Autodesk Inventor part; units mm, degrees
ref_plane "Start Plane" through (0, 0, 0) normal (1, 0, 0) x (0, 1, 0)
ref_plane "XZ Plane" through (0, 0, 0) normal (0, 1, 0) x (-1, 0, 0)
ref_plane "XY Plane" through (0, 0, 0) normal (0, 0, 1) x (1, 0, 0)
sketch "Main Sketch" plane through (0, 0, 0) normal (0, 0, 1) x (1, 0, 0)
  line L0 (0, 0) -> (40, 0)
  line L1 (0, 3) -> (0, 10)
  line L2 (40, 10) -> (40, 3)
  line L3 (0, 10) -> (40, 10)
  line L4 (12, 3) -> (12, 0)
  line L5 (0, 3) -> (12, 3)
  line L6 (28, 3) -> (28, 0)
  line L7 (40, 3) -> (28, 3)
  line L8 (12, 0) -> (28, 0)
  dimension "d3" = 20
  dimension "d4" = 6
  dimension "d5" = 6
revolve "Revolution1" add sketch "Main Sketch" angle 360 about axis through (0, 0, 0) along (1, 0, 0)
equation "\"Length\" = 40"
properties part number "Shaft" material "Aluminum 6061"
Check sheet for the modelled part. Datum: model origin and axes. Units: mm. A direction names the side the tool comes from. Coordinates: 2 decimals unless noted, no trailing zeros. Write each loop counter-clockwise with the first axis right and the second up, starting at its lowest first coordinate (ties: lowest second). Pieces come first, ordered by that corner, then holes. Notation, with made-up numbers: M 50,59 L 69,59 A9 ccw 69,68 Z; hole C 87.25,31.5 d6. An arc over 180 degrees is marked long. Answer as CSV lines item,"result".
Q1. Set-up check for faces 5 (the face through (12, 0, 0)), 6 (the face through (0, 2.1, 2.4)), 7 (the face through (28, 0, 0)): record each of +Z, -Z, +X, -X, +Y, -Y from which the full face is reachable in a straight line by a thin tool's end or side.
Check result:
face 5,"-X"
face 6,"+Z, -Z, -X, +Y, -Y"
face 7,"+X"
Q2. Mould release check, pull along Y, two halves, no side actions. Record for faces 1 (the face through (40, 2.1, 2.4)), 2 (the face through (20.28, -2.17, -9.76)), 3 (the face through (34, -3, 0)), 4 (the face through (6, -3, 0)): released by +Y, released by -Y, zero draft, split by the parting line, or undercut.
Check result:
face 1,"zero draft"
face 2,"split by the parting line"
face 3,"undercut"
face 4,"undercut"
Q3. Cross-section at C-C (x = 27.5). Record the boundary of the cut face in (y, z).
Check result:
outline,"C 0,0 d20"
Q4. Cross-section at D-D (x = 2). Record the boundary of the cut face in (y, z), then the cut area to 3 significant figures.
Check result:
outline,"C 0,0 d20; hole C 0,0 d6"
area,"286 mm^2"
Q5. Cross-section at A-A (z = 0). Record the boundary of the cut face in (x, y), then the cut area to 3 significant figures.
Check result:
outline,"M 0,-10 L 40,-10 L 40,-3 L 28,-3 L 28,3 L 40,3 L 40,10 L 0,10 L 0,3 L 12,3 L 12,-3 L 0,-3 Z"
area,"656 mm^2"
Q6. Go/stop test with flat-tipped pins: pin 1 (5 mm diameter, centred on x = 11.5, z = -2, fed in from -Y); pin 2 (1.8 mm diameter, centred on y = -0.5, z = -1.5, fed in from +X); pin 3 (5 mm diameter, centred on x = 7, z = -5.5, fed in from +Y); pin 4 (5 mm diameter, centred on x = 15.5, z = 6.5, fed in from +Y). Record where each tip stops, or that it passes through.
Check result:
pin 1,"y = -10"
pin 2,"x = 28"
pin 3,"y = 9.54"
pin 4,"y = 9.17"
Q7. Material ranges on probe 1 along Z at (x, y) = (4.75, 0); probe 2 along Z at (x, y) = (18, -0.5); probe 3 along Z at (x, y) = (12, 6), recorded low to high. Write a range as from..to.
Check result:
probe 1,"-10..-3, 3..10"
probe 2,"-9.99..9.99"
probe 3,"-8..8"
